Build history of the part. All positions in model axes, mm. A direction names the side the tool comes from. Give positions to 0.01 mm unless a question says otherwise; leave off trailing zeros. Loops run counter-clockwise (first coordinate to the right, second up) from the corner with the lowest first, then second, coordinate; pieces in that order, holes last.
1) Band-saw the part on A-A on x = 3.25. List the corners of the cut face in (y, z), then the cut area to 3 significant figures.
2) 3-axis set-ups, long thin cutter, end or side, ignore diameter. For faces 5 (the cylindrical face through (6.23, -0.01, -2.85)), 6 (the flat face through (-6.5, -0.5, -1.8)): which of +Z, -Z, +X, -X, +Y, -Y reach the whole face in a straight line?
3) Band-saw the part on B-B on y = -0.2. State how many separate pieces and enclosed holes the cut face has, then the cut area to 3 significant figures.
4) Two-plate mould, pull along X, no slides. Class faces 1 (the flat face through (-6.5, 0.5, -1.8)), 2 (the cylindrical face through (6.964, -0.007, -5.13)), 3 (the cylindrical face through (5.947, -0.007, 3.659)), 4 (the cylindrical face through (6.21, -0.01, 2.86)): +X half, -X half, draft (parallel to the pull), parting line (faces both ways), or undercut.
5) Wall check: line 1 (X direction, y = 0.35, z = -3.8); line 2 (Z direction, x = 0, y = 0.2); line 3 (Z direction, x = -1.5, y = 0.25). Give the ranges that are in metal, low to high.
6) Band-saw the part on D-D on x = 1.5. List the corners of the cut face in (y, z), then the cut area to 3 significant figures.
7) Band-saw the part on C-C on z = 0. List the corners of the cut face in (x, y), then the cut area to 3 significant figures.
```python
from build123d import *

# Parameters (mm, degrees)
BOSS_EXTRUDE1_DEPTH      = 0.5
BOSS_EXTRUDE1_DEPTH_BACK = 0.5
SKETCH3_R                = 0.65


with BuildPart() as part:
    # Sketch3 → Boss-Extrude1 (new, two sides: drawn at the far end of the back side and taken through both)
    with BuildSketch(Plane(origin=(0, 0, 0), x_dir=(1, 0, 0), z_dir=(0, 1, 0)).offset(-BOSS_EXTRUDE1_DEPTH_BACK)):
        with BuildLine():
            Line((4.921075662, 6.151466642), (5.415516704, 6.356270827))
            ThreePointArc((5.415516704, 6.356270827), (5.713132029, 6.387250398), (5.979333, 6.25060612))
            ThreePointArc((5.979333, 6.25060612), (6.97684177, 5.113333445), (7.760966936, 3.819671741))
            ThreePointArc((7.760966936, 3.819671741), (7.78120317, 3.402716753), (7.490834393, 3.102805199))
            Line((7.490834393, 3.102805199), (6.954149928, 2.880503215))
            ThreePointArc((6.954149928, 2.880503215), (6.218652108, 2.855007785), (5.647075885, 3.318589151))
            ThreePointArc((5.647075885, 3.318589151), (-6.55, 0), (5.647075885, -3.318589151))
            ThreePointArc((5.647075885, -3.318589151), (6.218652108, -2.855007785), (6.954149928, -2.880503215))
            Line((6.954149928, -2.880503215), (7.490834393, -3.102805199))
            ThreePointArc((7.490834393, -3.102805199), (7.78120317, -3.402716753), (7.760966936, -3.819671741))
            ThreePointArc((7.760966936, -3.819671741), (6.97684177, -5.113333445), (5.979333, -6.25060612))
            ThreePointArc((5.979333, -6.25060612), (5.713132029, -6.387250398), (5.415516704, -6.356270827))
            Line((5.415516704, -6.356270827), (4.921075662, -6.151466642))
            ThreePointArc((4.921075662, -6.151466642), (4.645102726, -6.116897415), (4.390197066, -6.228159258))
            ThreePointArc((4.390197066, -6.228159258), (-8.65, 0), (4.390197066, 6.228159258))
            ThreePointArc((4.390197066, 6.228159258), (4.645102726, 6.116897415), (4.921075662, 6.151466642))
        make_face()
        with Locations(Location((6.581793069, -3.8, 0), (0, 0, 270))):
            Circle(SKETCH3_R, mode=Mode.SUBTRACT)
        with Locations(Location((6.581793069, 3.8, 0), (0, 0, 270))):
            Circle(SKETCH3_R, mode=Mode.SUBTRACT)
    extrude(amount=BOSS_EXTRUDE1_DEPTH + BOSS_EXTRUDE1_DEPTH_BACK)


solid = part.part
```
Findings below:
1. outline: (-0.5, -7) - (0.5, -7) - (0.5, -5.69) - (-0.5, -5.69) - close; (-0.5, 5.69) - (0.5, 5.69) - (0.5, 7) - (-0.5, 7) - close
1. area: 2.62 mm2
2. face 5: +Y, -Y
2. face 6: +Z, -Z, +X, -X, -Y
3. separate pieces: 1
3. enclosed holes: 2
3. area: 68.1 mm2
4. face 1: draft
4. face 2: +X half
4. face 3: undercut
4. face 4: undercut
5. line 1: x = -7.69 to -5.34, 5.34 to 5.93, 7.23 to 7.77
5. line 2: z = -7.98 to -6.55, 6.55 to 7.98
5. line 3: z = -7.96 to -6.38, 6.38 to 7.96
6. outline: (-0.5, -7.72) - (0.5, -7.72) - (0.5, -6.38) - (-0.5, -6.38) - close; (-0.5, 6.38) - (0.5, 6.38) - (0.5, 7.72) - (-0.5, 7.72) - close
6. area: 2.68 mm2
7. outline: (-8.65, -0.5) - (-6.55, -0.5) - (-6.55, 0.5) - (-8.65, 0.5) - close
7. area: 2.10 mm2
